from build123d import *

# Parameters (mm, degrees)
SKETCH1_W               = 323
SKETCH1_H               = 120
BOSS_EXTRUDE1_DEPTH     = 3
SKETCH2_W               = 313
SKETCH2_H               = 110
SKETCH2_W_2             = 303
SKETCH2_H_2             = 100
CUT_EXTRUDE2_DEPTH      = 1.5
SKETCH2_4_W             = 303
SKETCH2_4_H             = 100
CUT_EXTRUDE3_DEPTH      = 1
CUT_EXTRUDE3_DEPTH_BACK = 4
SKETCH3_W               = 323
SKETCH3_H               = 2.051483501
BOSS_EXTRUDE2_DEPTH     = 3


with BuildPart() as part:
    # Sketch1 → Boss-Extrude1 (new body)
    with BuildSketch(Plane(origin=(0, 0, 0), x_dir=(1, 0, 0), z_dir=(0, 1, 0))):
        Rectangle(SKETCH1_W, SKETCH1_H)
    extrude(amount=BOSS_EXTRUDE1_DEPTH)

    # Sketch2 → Cut-Extrude2 (cut)
    with BuildSketch(Plane(origin=(0, 3, 0), x_dir=(1, 0, 0), z_dir=(0, 1, 0))):
        Rectangle(SKETCH2_W, SKETCH2_H)
        Rectangle(SKETCH2_W_2, SKETCH2_H_2, mode=Mode.SUBTRACT)
    extrude(amount=-CUT_EXTRUDE2_DEPTH, mode=Mode.SUBTRACT)

    # Sketch2_4 → Cut-Extrude3 (cut, two sides)
    with BuildSketch(Plane(origin=(0, 3, 0), x_dir=(1, 0, 0), z_dir=(0, 1, 0))) as cut_extrude3_sk:
        Rectangle(SKETCH2_4_W, SKETCH2_4_H)
    extrude(amount=CUT_EXTRUDE3_DEPTH, mode=Mode.SUBTRACT)
    extrude(cut_extrude3_sk.sketch, amount=-CUT_EXTRUDE3_DEPTH_BACK, mode=Mode.SUBTRACT)

    # Sketch3 → Boss-Extrude2 (add)
    with BuildSketch(Plane(origin=(0, 3, 0), x_dir=(1, 0, 0), z_dir=(0, 1, 0))):
        with Locations((0, -61.025741751)):
            Rectangle(SKETCH3_W, SKETCH3_H)
    extrude(amount=-BOSS_EXTRUDE2_DEPTH)


solid = part.part
Here's how the part is built. I have some questions about the finished solid (model axes, mm). Give positions to 0.01 mm unless a question says otherwise; leave off trailing zeros. Order: outer loops, then holes, each group sorted by start corner. A loop starts at its lowest first (then second) coordinate and runs counter-clockwise, first axis right, second up. Notation, with made-up numbers: M 79.25,-10.5 L 103.25,-10.5 A16 cw 103.25,2.5 Z; hole C 53,69 d1. An arc over 180 degrees is marked long. Answer as a JSON object with one key per item and string values. Group by question number.
1) Suppose I cut it at C-C, the plane y = 2.3. Write out the boundary of the cut face in (x, z).
2) We'd pull the mould along X, two halves only. Please class faces 1 (the flat face through (-1, 1.5, -53)), 2 (the flat face through (-1, 3, -58)): pulls with the +X half, pulls with the -X half, needs draft (parallel to the pull), parting line crosses it, or undercut.
3) Please list where these lines run through material, in increasing order: L1, parallel to X at y = 0.95, z = 33; L2, parallel to Z at x = 76.5, y = 2.55; L3, parallel to X at y = 1.7, z = -50.5. Write a range as [from, to].
4) Suppose I cut it at B-B, the plane x = -118. Write out the boundary of the cut face in (y, z).
5) Suppose I cut it at A-A, the plane z = -3. Write out the boundary of the cut face in (x, y), plus the area to 3 significant figures.
Results found:
{
 "1": {"outline": "M -161.5,-60 L 161.5,-60 L 161.5,62.05 L -161.5,62.05 Z; hole M -156.5,-55 L 156.5,-55 L 156.5,55 L -156.5,55 Z"},
 "2": {"face 1": "undercut", "face 2": "needs draft"},
 "3": {"L1": "[-161.5, -151.5], [151.5, 161.5]", "L2": "[-60, -55], [55, 62.05]", "L3": "[-161.5, -156.5], [156.5, 161.5]"},
 "4": {"outline": "M 0,-60 L 3,-60 L 3,-55 L 1.5,-55 L 1.5,-50 L 0,-50 Z; M 0,50 L 1.5,50 L 1.5,55 L 3,55 L 3,62.05 L 0,62.05 Z"},
 "5": {"outline": "M -161.5,0 L -151.5,0 L -151.5,1.5 L -156.5,1.5 L -156.5,3 L -161.5,3 Z; M 151.5,0 L 161.5,0 L 161.5,3 L 156.5,3 L 156.5,1.5 L 151.5,1.5 Z", "area": "45.0 mm²"}
}
